Geometry check sheet. Reference: the model listing, model coordinates, mm. Give positions to 0.01 mm unless a question says otherwise; leave off trailing zeros. Order: outer loops, then holes, each group sorted by start corner. A loop starts at its lowest first (then second) coordinate and runs counter-clockwise, first axis right, second up. Notation, with made-up numbers: M 18,31.5 L 64,31.5 A31 cw 64,62.5 Z; hole C -7,48.5 d10. An arc over 180 degrees is marked long. Answer as CSV lines item,"result". Start each with the question number.
Q1. Section check B-B, the plane x = 0. Record the boundary of the cut face in (y, z), then the cut area to 3 significant figures.
Q2. Go/stop test with flat-tipped pins: pin 1 (18 mm diameter, centred on x = 0, y = -25, fed in from +Z); pin 2 (4 mm diameter, centred on x = -6.5, y = -15.5, fed in from -Z); pin 3 (8 mm diameter, centred on x = 12.5, z = 15, fed in from +Y). Record where each tip stops, or that it passes through.
Q3. Mould release check, pull along Y, two halves, no side actions. Record for faces 1 (the flat face through (0, 0, 15)), 2 (the flat face through (-20, -25, 10)), 3 (the cylindrical face through (9.54, -22, 14.15)), 4 (the flat face through (0, -50, 15)): +Y half, -Y half, draft (parallel to the pull), parting line (faces both ways), or undercut.
Q4. Section check A-A, the plane y = -25. Record the boundary of the cut face in (x, z).
Q5. Section check D-D, the plane y = -5. Record the boundary of the cut face in (x, z), then the cut area to 3 significant figures.
Q6. Section check C-C, the plane z = 14.25. Record the boundary of the cut face in (x, y).
Q7. Thickness scan on line 1 (Y direction, x = 0, z = 14); line 2 (X direction, y = -25, z = 13.5); line 3 (X direction, y = -48, z = 1). Record the ranges inside material, lowest first.
```python
from build123d import *

# Parameters (mm, degrees)
F0_W     = 40
F0_H     = 20
F1_DEPTH = 50
F2_R     = 24
F3_DEPTH = 50.001
F4_R     = 10
F5_DEPTH = 19.913378


with BuildPart() as f1:
    # F0 (on Front) → F1 (new body)
    with BuildSketch(Plane.XZ):
        with Locations((0, 9.912378)):
            Rectangle(F0_W, F0_H)
    extrude(amount=F1_DEPTH)

    # F2 (on Front) → F3 (cut, through all)
    with BuildSketch(Plane.XZ):
        with Locations((0, -13.266499)):
            Circle(F2_R)
    extrude(amount=F3_DEPTH, mode=Mode.SUBTRACT)

    # F4 (on Top) → F5 (cut, through all)
    with BuildSketch(Plane.XY):
        with Locations((0, -25)):
            Circle(F4_R)
    extrude(amount=F5_DEPTH, mode=Mode.SUBTRACT)


solid = f1.part
```
Answer block:
1,outline,"M -50,10.73 L -35,10.73 L -35,19.91 L -50,19.91 Z; M -15,10.73 L 0,10.73 L 0,19.91 L -15,19.91 Z"
1,area,"275 mm2"
2,pin 1,"passes through"
2,pin 2,"stops at z = 9.18"
2,pin 3,"stops at y = 0"
3,face 1,"+Y half"
3,face 2,"draft"
3,face 3,"undercut"
3,face 4,"-Y half"
4,outline,"M -20,0 A24 cw -10,8.55 L -10,19.91 L -20,19.91 Z; M 10,8.55 A24 cw 20,0 L 20,19.91 L 10,19.91 Z"
5,outline,"M -20,0 A24 cw 20,0 L 20,19.91 L -20,19.91 Z"
5,area,"494 mm2"
6,outline,"M -20,-50 L 20,-50 L 20,0 L -20,0 Z; hole C 0,-25 d20"
7,line 1,"y = -50 to -35, -15 to 0"
7,line 2,"x = -20 to -10, 10 to 20"
7,line 3,"x = -20 to -19.3, 19.3 to 20"
